from build123d import *

# Parameters (mm, degrees)
SKETCH_1_W          = 250
SKETCH_1_H          = 120
EXTRUDE_1_DEPTH     = 100
SKETCH_2_W          = 3
SKETCH_2_H          = 141.063947636
SKETCH_2_W_2        = 4.187427017
CUT_EXTRUDE_1_DEPTH = 10
SKETCH_3_W          = 2.606673318
SKETCH_3_H          = 138.805354188
SKETCH_3_W_2        = 4.561678307
SKETCH_3_W_3        = 2.389450542
CUT_EXTRUDE_2_DEPTH = 10


with BuildPart() as part:
    # 스케치1 → 보스-돌출1 (new body)
    with BuildSketch(Plane.XY):
        with Locations((45, 0)):
            Rectangle(SKETCH_1_W, SKETCH_1_H)
    extrude(amount=EXTRUDE_1_DEPTH)

    # 스케치2 → 컷-돌출1 (cut)
    with BuildSketch(Plane(origin=(170, 0, 0), x_dir=(0, 0, -1), z_dir=(1, 0, 0))):
        with Locations((-46.296564822, 2.74799898)):
            Rectangle(SKETCH_2_W, SKETCH_2_H)
        with Locations((-29.546856754, 2.74799898)):
            Rectangle(SKETCH_2_W, SKETCH_2_H)
        with Locations((-12.988577744, 2.74799898)):
            Rectangle(SKETCH_2_W_2, SKETCH_2_H)
    extrude(amount=-CUT_EXTRUDE_1_DEPTH, mode=Mode.SUBTRACT)

    # 스케치3 → 컷-돌출2 (cut)
    with BuildSketch(Plane.ZY.offset(80)):
        with Locations((10.910436229, 0.546851797)):
            Rectangle(SKETCH_3_W, SKETCH_3_H)
        with Locations((31.220765833, 0.546851797)):
            Rectangle(SKETCH_3_W_2, SKETCH_3_H)
        with Locations((49.033033506, 0.546851797)):
            Rectangle(SKETCH_3_W_3, SKETCH_3_H)
    extrude(amount=-CUT_EXTRUDE_2_DEPTH, mode=Mode.SUBTRACT)


solid = part.part
Model file for the job. Use its own axes, mm. A direction names the side the tool comes from. Give positions to 0.01 mm unless a question says otherwise; leave off trailing zeros. One line per item, written item: value. Start each with the question number.
Q1. Drop flat-ended pins along their axis: pin 1 Ø1.2 at (y, z) = (17.5, 48.5) entering from -X; pin 2 Ø1.3 at (y, z) = (14, 13) entering from +X. Give the stop position or say it passes through.
Q2. Two-plate mould, pull along Z, no slides. Class faces 4 (the flat face through (-75, -1, 12.214)), 5 (the flat face through (170, -1, 38)), 6 (the flat face through (43, 1, 0)): +Z half, -Z half, draft (parallel to the pull), parting line (faces both ways), or undercut.
Q3. 3-axis set-ups, long thin cutter, end or side, ignore diameter. For faces 1 (the flat face through (170, -1, 5)), 2 (the flat face through (-75, -1, 28.94)), 3 (the flat face through (165, -1, 28.047)): which of +Z, -Z, +X, -X, +Y, -Y reach the whole face in a straight line?
Q4. Probe probe 1 along X at (y, z) = (50, 46.5). List the from-to ranges inside material, lowest first. Write a range as [from, to].
Output values:
1. pin 1: stops at x = -70
1. pin 2: stops at x = 160
2. face 4: undercut
2. face 5: draft
2. face 6: -Z half
3. face 1: +Z, -Z, +X, +Y, -Y
3. face 2: -X, +Y, -Y
3. face 3: +X, +Y, -Y
4. probe 1: x = [-80, 160]
